Verification items for the finished model (mm, model axes). A direction names the side the tool comes from. Give positions to 0.01 mm unless a question says otherwise; leave off trailing zeros. Write each loop counter-clockwise with the first axis right and the second up, starting at its lowest first coordinate (ties: lowest second). Pieces come first, ordered by that corner, then holes. Notation, with made-up numbers: (53.5, -13) -> (61.5, -13) arc R14 cw to (61.5, 7) -> close; hole circle Ø9 at (81, -28.5). An arc over 180 degrees is marked (long way). Answer as CSV lines item,"result". Start each with the question number.
1) Sectioned sample at D-D on x = 15. Record the cut outline in (y, z) (3 decimals).
2) Sectioned sample at B-B on x = -4. Record the cut outline in (y, z).
3) Tool access check on faces 1 (the flat face through (-14, 11.875, 0)), 2 (the flat face through (-2.875, 13, -14)), 3 (the cylindrical face through (-1.21, 10.92, 12.42)). Record the directions out of +Z, -Z, +X, -X, +Y, -Y that give a thin tool (end or side, any length) a straight path to the whole face; none if there is none.
4) Sectioned sample at C-C on z = -14.5. Record the cut outline in (x, y) (3 decimals), and give its area (3 significant figures).
5) Mould release check, pull along X, two halves, no side actions. Record for faces 4 (the flat face through (9.6, 13.27, -1.42)), 5 (the flat face through (-9.622, 13.231, 1.458)), 6 (the flat face through (0, 8, -6.5)), 7 (the flat face through (8, 16.5, 0)): released by +X, released by -X, zero draft, split by the parting line, or undercut.
6) Sectioned sample at A-A on y = 13.5. Record the cut outline in (x, z) (3 decimals).
7) Gauge pin test, flat ends, axial feed: pin 1 Ø2 at (x, y) = (4, 3) entering from +Z; pin 2 Ø0.6 at (x, z) = (11.5, -0.5) entering from +Y; pin 3 Ø4 at (y, z) = (12.5, -1.5) entering from +X; pin 4 Ø3 at (y, z) = (3.5, 12.5) entering from -X. Record the tip position at first contact, or that the pin passes through.
8) Material ranges on L1, parallel to Y at x = 0, z = -9 (3 decimals); L2, parallel to Z at x = 1, y = 11.5; L3, parallel to Y at x = -2.5, z = -14 (3 decimals), recorded low to high.
```python
from build123d import *

# Parameters (mm, degrees)
SKETCH1_R                      = 12
SKETCH1_W                      = 13
SKETCH1_H                      = 13
BOSS_EXTRUDE1_DEPTH            = 10
SKETCH2_R                      = 17.5
BOSS_EXTRUDE2_DEPTH            = 6.5
CUT_EXTRUDE1_REACH             = 28.693
SKETCH3_R                      = 1.25
CUT_EXTRUDE2_DEPTH             = 30.744747435
CUT_EXTRUDE2_DEPTH_BACK        = 30.744747435
SKETCH4_R                      = 1.5
CUT_EXTRUDE3_REACH             = 28.693
SKETCH6_W                      = 13
SKETCH6_H                      = 13
CUT_EXTRUDE3_DIRECTION_2_DEPTH = 10
SKETCH8_W                      = 5.75
SKETCH8_H                      = 2.75
CUT_EXTRUDE4_DEPTH             = 5
CUT_EXTRUDE5_DEPTH             = 2.75
CIRPATTERN1_START              = 11.875
CIRPATTERN1_OUTLINE_R          = 1.25
CIRPATTERN1_DEPTH              = 2.75


# Read off the part's stored shape, not the designer's step: CirPattern1
with BuildPart() as part:
    # Sketch1 → Boss-Extrude1 (new body)
    with BuildSketch(Plane(origin=(0, 0, 0), x_dir=(1, 0, 0), z_dir=(0, 1, 0))):
        with Locations(Location((0, 0, 0), (0, 0, 270))):
            Circle(SKETCH1_R)
        Rectangle(SKETCH1_W, SKETCH1_H, mode=Mode.SUBTRACT)
    extrude(amount=BOSS_EXTRUDE1_DEPTH)

    # Sketch2 → Boss-Extrude2 (add)
    with BuildSketch(Plane(origin=(0, 10, 0), x_dir=(1, 0, 0), z_dir=(0, 1, 0))):
        with Locations(Location((0, 0, 0), (0, 0, 90))):
            Circle(SKETCH2_R)
    extrude(amount=BOSS_EXTRUDE2_DEPTH)

    # Sketch3 → Cut-Extrude1 (cut, up to next)
    with BuildSketch(Plane.XZ.offset(-10), mode=Mode.PRIVATE) as cut_extrude1_sk1:
        with Locations(Location((12.1, 0, 0), (0, 0, 262.453989537))):
            Circle(SKETCH3_R)
    cut_extrude1_tool1 = extrude(cut_extrude1_sk1.sketch, amount=-CUT_EXTRUDE1_REACH, mode=Mode.PRIVATE) & part.part
    # Sketch3 → Cut-Extrude1 (cut, up to next)
    with BuildSketch(Plane.XZ.offset(-10), mode=Mode.PRIVATE) as cut_extrude1_sk2:
        with Locations(Location((0, -12.1, 0), (0, 0, 172.453989537))):
            Circle(SKETCH3_R)
    cut_extrude1_tool2 = extrude(cut_extrude1_sk2.sketch, amount=-CUT_EXTRUDE1_REACH, mode=Mode.PRIVATE) & part.part
    # Sketch3 → Cut-Extrude1 (cut, up to next)
    with BuildSketch(Plane.XZ.offset(-10), mode=Mode.PRIVATE) as cut_extrude1_sk3:
        with Locations(Location((-12.1, 0, 0), (0, 0, 277.546010463))):
            Circle(SKETCH3_R)
    cut_extrude1_tool3 = extrude(cut_extrude1_sk3.sketch, amount=-CUT_EXTRUDE1_REACH, mode=Mode.PRIVATE) & part.part
    # Sketch3 → Cut-Extrude1 (cut, up to next)
    with BuildSketch(Plane.XZ.offset(-10), mode=Mode.PRIVATE) as cut_extrude1_sk4:
        with Locations(Location((0, 12.1, 0), (0, 0, 187.546010463))):
            Circle(SKETCH3_R)
    cut_extrude1_tool4 = extrude(cut_extrude1_sk4.sketch, amount=-CUT_EXTRUDE1_REACH, mode=Mode.PRIVATE) & part.part
    add(cut_extrude1_tool1.solids().sort_by_distance((12.1, 10, 0))[0], mode=Mode.SUBTRACT)
    add(cut_extrude1_tool2.solids().sort_by_distance((0, 10, -12.1))[0], mode=Mode.SUBTRACT)
    add(cut_extrude1_tool3.solids().sort_by_distance((-12.1, 10, 0))[0], mode=Mode.SUBTRACT)
    add(cut_extrude1_tool4.solids().sort_by_distance((0, 10, 12.1))[0], mode=Mode.SUBTRACT)

    # Sketch4 → Cut-Extrude2 (cut, two sides: drawn at the far end of the back side and taken through both)
    with BuildSketch(Plane.XY.offset(-CUT_EXTRUDE2_DEPTH_BACK)):
        with Locations((0, 4.916404418)):
            Circle(SKETCH4_R)
    extrude(amount=CUT_EXTRUDE2_DEPTH + CUT_EXTRUDE2_DEPTH_BACK, mode=Mode.SUBTRACT)

    # Sketch6 → Cut-Extrude3 (cut, up to next)
    with BuildSketch(Plane(origin=(0, 10, 0), x_dir=(-1, 0, 0), z_dir=(0, -1, 0)), mode=Mode.PRIVATE) as cut_extrude3_sk1:
        Rectangle(SKETCH6_W, SKETCH6_H)
    cut_extrude3_tool1 = extrude(cut_extrude3_sk1.sketch, amount=-CUT_EXTRUDE3_REACH, mode=Mode.PRIVATE) & part.part
    add(cut_extrude3_tool1.solids().sort_by_distance((0, 10, 0))[0], mode=Mode.SUBTRACT)

    # Sketch6 → Cut-Extrude3 direction 2 (cut)
    with BuildSketch(Plane(origin=(0, 10, 0), x_dir=(-1, 0, 0), z_dir=(0, -1, 0))):
        Rectangle(SKETCH6_W, SKETCH6_H)
    extrude(amount=CUT_EXTRUDE3_DIRECTION_2_DEPTH, mode=Mode.SUBTRACT)

    # Sketch8 → Cut-Extrude4 (cut)
    with BuildSketch(Plane(origin=(17.5, 0, 0), x_dir=(0, 0, -1), z_dir=(1, 0, 0))):
        with Locations((0, 13.25)):
            Rectangle(SKETCH8_W, SKETCH8_H)
    extrude(amount=-CUT_EXTRUDE4_DEPTH, mode=Mode.SUBTRACT)

    # Sketch9 → Cut-Extrude5 (cut)
    with BuildSketch(Plane.XZ.offset(-14.625)):
        Polygon((15.419764048, 0), (13.759882024, 2.875), (10.440117976, 2.875), (8.780235952, 0), (10.440117976, -2.875), (13.759882024, -2.875), align=None)
    extrude(amount=CUT_EXTRUDE5_DEPTH, mode=Mode.SUBTRACT)

    # CirPattern1 outline → CirPattern1 (cut)
    # profile 1 of 3: a face of its own
    with BuildSketch(Plane(origin=(0, 0, 0), x_dir=(1, 0, 0), z_dir=(0, 1, 0)).offset(CIRPATTERN1_START)):
        with BuildLine():
            Line((-8.780235952, 0), (-10.440117976, 2.875))
            Line((-10.440117976, 2.875), (-17.26222393, 2.875))
            ThreePointArc((-17.26222393, 2.875), (-17.5, 0), (-17.26222393, -2.875))
            Line((-17.26222393, -2.875), (-10.440117976, -2.875))
            Line((-10.440117976, -2.875), (-8.780235952, 0))
        make_face()
        with Locations((-12.1, 0)):
            Circle(CIRPATTERN1_OUTLINE_R, mode=Mode.SUBTRACT)
    # profile 2 of 3: a face of its own
    with BuildSketch(Plane(origin=(0, 0, 0), x_dir=(1, 0, 0), z_dir=(0, 1, 0)).offset(CIRPATTERN1_START)):
        with BuildLine():
            ThreePointArc((2.875, 17.26222393), (0, 17.5), (-2.875, 17.26222393))
            Line((-2.875, 17.26222393), (-2.875, 10.440117976))
            Line((-2.875, 10.440117976), (0, 8.780235952))
            Line((0, 8.780235952), (2.875, 10.440117976))
            Line((2.875, 10.440117976), (2.875, 17.26222393))
        make_face()
        with Locations((0, 12.1)):
            Circle(CIRPATTERN1_OUTLINE_R, mode=Mode.SUBTRACT)
    # profile 3 of 3: a face of its own
    with BuildSketch(Plane(origin=(0, 0, 0), x_dir=(1, 0, 0), z_dir=(0, 1, 0)).offset(CIRPATTERN1_START)):
        with BuildLine():
            Line((-2.875, -10.440117976), (-2.875, -17.26222393))
            ThreePointArc((-2.875, -17.26222393), (0, -17.5), (2.875, -17.26222393))
            Line((2.875, -17.26222393), (2.875, -10.440117976))
            Line((2.875, -10.440117976), (0, -8.780235952))
            Line((0, -8.780235952), (-2.875, -10.440117976))
        make_face()
        with Locations((0, -12.1)):
            Circle(CIRPATTERN1_OUTLINE_R, mode=Mode.SUBTRACT)
    extrude(amount=CIRPATTERN1_DEPTH, mode=Mode.SUBTRACT)


solid = part.part
```
Ans:
1,outline,"(10, -9.014) -> (16.5, -9.014) -> (16.5, 9.014) -> (10, 9.014) -> close; hole (11.875, -2.875) -> (14.625, -2.875) -> (14.625, 2.875) -> (11.875, 2.875) -> close"
2,outline,"(0, -11.31) -> (10, -11.31) -> (10, -17.04) -> (16.5, -17.04) -> (16.5, -6.5) -> (0, -6.5) -> close; (0, 6.5) -> (16.5, 6.5) -> (16.5, 17.04) -> (10, 17.04) -> (10, 11.31) -> (0, 11.31) -> close"
3,face 1,"-X"
3,face 2,"-Z"
3,face 3,"+Y"
4,outline,"(-9.798, 10) -> (9.798, 10) -> (9.798, 16.5) -> (-9.798, 16.5) -> close; hole (-2.875, 11.875) -> (2.875, 11.875) -> (2.875, 14.625) -> (-2.875, 14.625) -> close"
4,area,"112 mm²"
5,face 4,"released by +X"
5,face 5,"released by -X"
5,face 6,"undercut"
5,face 7,"zero draft"
6,outline,"(-17.262, -2.875) arc R17.5 ccw to (-2.875, -17.262) -> (-2.875, -10.44) -> (0, -8.78) -> (2.875, -10.44) -> (2.875, -17.262) arc R17.5 ccw to (17.262, -2.875) -> (10.44, -2.875) -> (8.78, 0) -> (10.44, 2.875) -> (17.262, 2.875) arc R17.5 ccw to (2.875, 17.262) -> (2.875, 10.44) -> (0, 8.78) -> (-2.875, 10.44) -> (-2.875, 17.262) arc R17.5 ccw to (-17.262, 2.875) -> (-10.44, 2.875) -> (-8.78, 0) -> (-10.44, -2.875) -> close; hole (-6.5, -6.5) -> (6.5, -6.5) -> (6.5, 6.5) -> (-6.5, 6.5) -> close"
7,pin 1,"stops at z = 11.62"
7,pin 2,"stops at y = 10"
7,pin 3,"stops at x = 17.5"
7,pin 4,"stops at x = -4.8"
8,L1,"y = 0 to 3.416, 6.416 to 11.875, 14.625 to 16.5"
8,L2,"z = -17.47 to -12.85, -11.35 to -6.5, 6.5 to 11.35, 12.85 to 17.47"
8,L3,"y = 10 to 11.875, 14.625 to 16.5"
